Geometry: see drawing. Coordinates: mm, zero at the bounding-box minimum. Round coordinates to 2 decimals unless told otherwise and drop trailing zeros. Loops run counter-clockwise (first coordinate to the right, second up) from the corner with the lowest first, then second, coordinate; pieces in that order, holes last. Notation, with made-up numbers: (38.25, 86.25) - (83.25, 86.25) arc R31 cw to (83.25, 112.25) - close; hole circle Ø8 at (26, -1). An arc over 180 degrees is marked (long way). Write item = value, one per line. Start each with the question number.
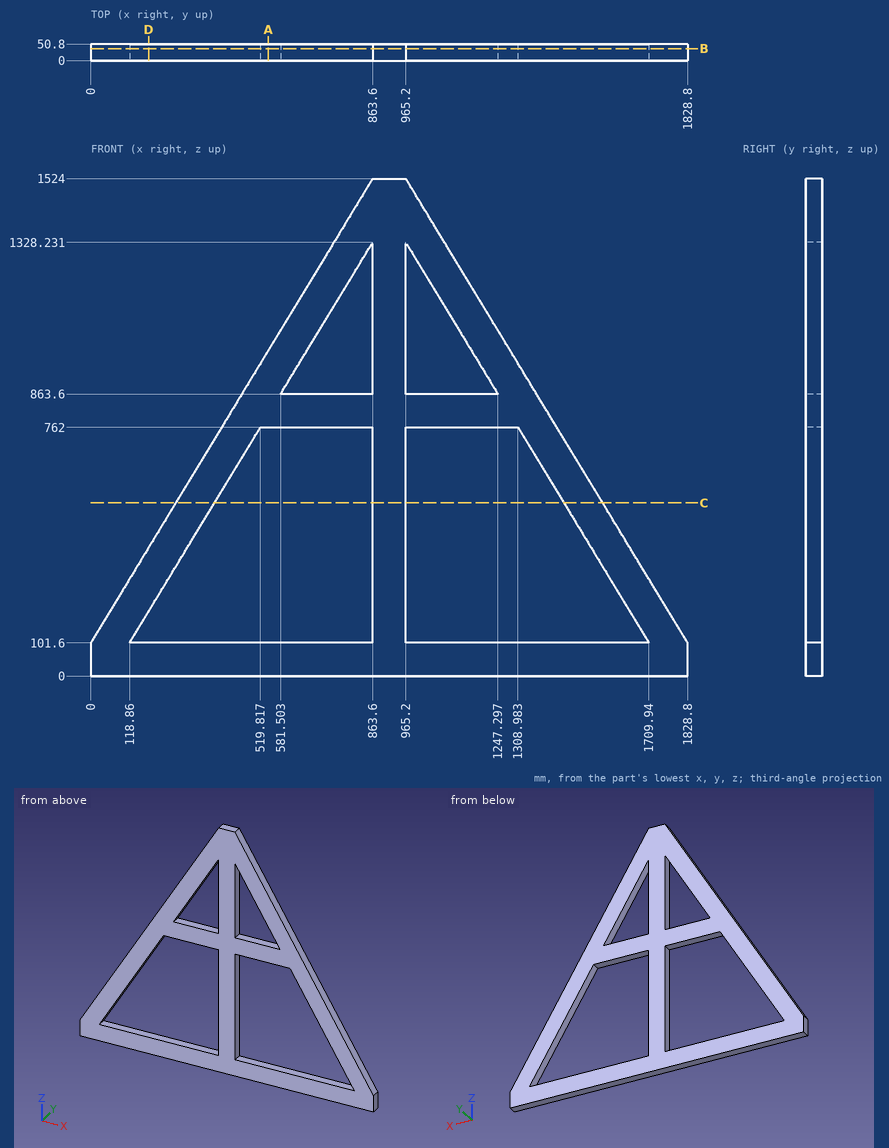
(1) Cut plane B-B (y = 37). Output: boundary loops of the cut face in (x, z).
(2) Material intervals for line 1 along X through (y, z) = (34.5, 1102.5); line 2 along Z through (x, y) = (1099.5, 36); line 3 along X through (y, z) = (31.5, 286), sorted ascending. Write a range as from..to.
(3) Cut plane A-A (x = 544). Output: boundary loops of the cut face in (y, z).
(4) Pin query (flat end, axial travel): P1, Ø12, axis at y = 10.5, z = 252, coming from the -X side; P2, Ø3, axis at y = 40, z = 399.5, coming from the -X side; P3, Ø15, axis at y = 31, z = 1098.5, coming from the -X side. Return the tip coordinate at first contact, or that it passes through.
(5) Cut plane C-C (z = 530.5). Output: boundary loops of the cut face in (x, y).
(6) Cut plane D-D (x = 177.5). Output: boundary loops of the cut face in (y, z).
Solution:
q1.outline = (0, 0) - (1828.8, 0) - (1828.8, 101.6) - (965.2, 1524) - (863.6, 1524) - (0, 101.6) - close; hole (118.86, 101.6) - (863.6, 101.6) - (863.6, 762) - (519.82, 762) - close; hole (581.5, 863.6) - (863.6, 863.6) - (863.6, 1328.23) - close; hole (965.2, 101.6) - (1709.94, 101.6) - (1308.98, 762) - (965.2, 762) - close; hole (965.2, 863.6) - (1247.3, 863.6) - (965.2, 1328.23) - close
q2.line_1 = 607.69..726.55, 863.6..965.2, 1102.25..1221.11
q2.line_2 = 0..101.6, 762..863.6, 1107.03..1302.8
q2.line_3 = 111.96..230.82, 863.6..965.2, 1597.98..1716.84
q3.outline = (0, 0) - (50.8, 0) - (50.8, 101.6) - (0, 101.6) - close; (0, 762) - (50.8, 762) - (50.8, 997.6) - (0, 997.6) - close
q4.P1 = 87.67
q4.P2 = 179.96
q4.P3 = 600.71
q5.outline = (260.4, 0) - (379.26, 0) - (379.26, 50.8) - (260.4, 50.8) - close; (863.6, 0) - (965.2, 0) - (965.2, 50.8) - (863.6, 50.8) - close; (1449.54, 0) - (1568.4, 0) - (1568.4, 50.8) - (1449.54, 50.8) - close
q6.outline = (0, 0) - (50.8, 0) - (50.8, 101.6) - (0, 101.6) - close; (0, 198.18) - (50.8, 198.18) - (50.8, 393.95) - (0, 393.95) - close
